```python
from build123d import *

# Parameters (mm, degrees)
F1_DEPTH = 10
F2_R     = 5
F3_DEPTH = 25
F4_R     = 5
F5_DEPTH = 10


with BuildPart() as f1:
    # F0 (on Top) → F1 (new body)
    with BuildSketch(Plane.XY):
        Polygon((0, 25), (0, 30), (-14.694631, 20.225425), (-17.633558, 24.27051), (-23.776413, 7.725425), (-28.531695, 9.27051), (-23.776413, -7.725425), (-28.531695, -9.27051), (-14.694631, -20.225425), (-17.633558, -24.27051), (0, -25), (0, -30), (14.694631, -20.225425), (17.633558, -24.27051), (23.776413, -7.725425), (28.531695, -9.27051), (23.776413, 7.725425), (28.531695, 9.27051), (14.694631, 20.225425), (17.633558, 24.27051), align=None)
    extrude(amount=F1_DEPTH)

    # F2 (on Top) → F3 (join)
    with BuildSketch(Plane.XY):
        Circle(F2_R)
    extrude(amount=F3_DEPTH)

    # F4 (on Top) → F5 (join)
    with BuildSketch(Plane.XY):
        Circle(F4_R)
    extrude(amount=F5_DEPTH)


solid = f1.part
```
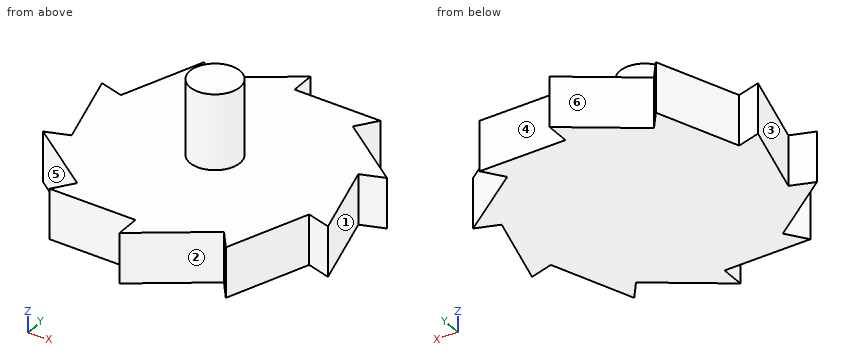
Verification items for the finished model (mm, model axes). Face numbers are marked on the shaded views. A direction names the side the tool comes from. Round coordinates to 2 decimals unless told otherwise and drop trailing zeros. Order: outer loops, then holes, each group sorted by start corner. A loop starts at its lowest first (then second) coordinate and runs counter-clockwise, first axis right, second up. Notation, with made-up numbers: (78, 30.5) - (106, 30.5) arc R27 ccw to (106, 49.5) - close; hole circle Ø11 at (-16, -20). An arc over 180 degrees is marked (long way). Use CSV: the item, a comma, the result in double quotes. Start each with the question number.
1) Go/stop test with flat-tipped pins: P1, Ø1.5, axis at y = -26.5, z = 4.5, coming from the -X side; P2, Ø3, axis at x = 11, z = 7, coming from the +Y side; P3, Ø10, axis at y = 3, z = 7, coming from the +X side. Record where each tip stops, or that it passes through.
2) Access from +Z, -Z, +X, -X, +Y, -Y to the whole of each face (thin tool, end or side, straight path). Record for the marked faces 1, 2 and 3.
3) Section check C-C, the plane y = 4. Record the cut outline in (x, z), plus the area to 3 significant figures.
4) Section check D-D, the plane x = 7. Record the cut outline in (y, z), plus the area to 3 significant figures.
5) Mould release check, pull along X, two halves, no side actions. Record for the marked faces 4, 5 and 6: +X half, -X half, draft (parallel to the pull), parting line (faces both ways), or undercut.
6) Section check B-B, the plane z = 9.25. Record the cut outline in (x, y), plus the area to 3 significant figures.
7) Section check A-A, the plane y = 23. Record the cut outline in (x, z), plus the area to 3 significant figures.
8) Thickness scan on L1, parallel to Z at x = 20.5, y = 7; L2, parallel to X at y = 22, z = 4.5; L3, parallel to Y at x = 17.5, z = 9. Record the ranges inside material, lowest first.
Answers:
1,P1,"stops at x = 0"
1,P2,"stops at y = 24.61"
1,P3,"stops at x = 26.5"
2,face 1,"+Z, -Z, +X"
2,face 2,"+Z, -Z, -Y"
2,face 3,"+Z, -Z, -X"
3,outline,"(-27.06, 0) - (24.82, 0) - (24.82, 10) - (3, 10) - (3, 25) - (-3, 25) - (-3, 10) - (-27.06, 10) - close"
3,area,"609 mm²"
4,outline,"(-25.34, 0) - (24.71, 0) - (24.71, 10) - (-25.34, 10) - close"
4,area,"501 mm²"
5,face 4,"+X half"
5,face 5,"-X half"
5,face 6,"undercut"
6,outline,"(-28.53, -9.27) - (-14.69, -20.23) - (-17.63, -24.27) - (0, -25) - (0, -30) - (14.69, -20.23) - (17.63, -24.27) - (23.78, -7.73) - (28.53, -9.27) - (23.78, 7.73) - (28.53, 9.27) - (14.69, 20.23) - (17.63, 24.27) - (0, 25) - (0, 30) - (-14.69, 20.23) - (-17.63, 24.27) - (-23.78, 7.73) - (-28.53, 9.27) - (-23.78, -7.73) - close"
6,area,"2,200 mm²"
7,outline,"(-18.11, 0) - (-16.71, 0) - (-16.71, 10) - (-18.11, 10) - close; (-10.52, 0) - (16.71, 0) - (16.71, 10) - (-10.52, 10) - close"
7,area,"286 mm²"
8,L1,"z = 0 to 10"
8,L2,"x = -18.48 to -15.98, -12.03 to 15.98"
8,L3,"y = -24.09 to 18, 24.09 to 24.28"
